from build123d import *

# Parameters (mm, degrees)
SKETCH_1_W           = 690
SKETCH_1_H           = 650
BOTTOM_PLATE_DEPTH   = 5
SKETCH_2_R           = 82.5
GRAB_CLEARANCE_DEPTH = 948.958332418
SKETCH_3_R           = 82.5
CUT_EXTRUDE_2_DEPTH  = 948.958332418
SKETCH_4_R           = 82.5
CUT_EXTRUDE_3_DEPTH  = 948.958332418
SKETCH_5_R           = 82.5
CUT_EXTRUDE_4_DEPTH  = 948.958332418


with BuildPart() as part:
    # 草图1 → Bottom_plate (new body)
    with BuildSketch(Plane.XY):
        with Locations((345, 325)):
            Rectangle(SKETCH_1_W, SKETCH_1_H)
    extrude(amount=BOTTOM_PLATE_DEPTH)

    # 草图2 → Grab_clearance (cut, through all)
    with BuildSketch(Plane.XY.offset(5)):
        with Locations((124, 92.5)):
            Circle(SKETCH_2_R)
    extrude(amount=-GRAB_CLEARANCE_DEPTH, mode=Mode.SUBTRACT)

    # 草图3 → 切除-拉伸2 (cut, through all)
    with BuildSketch(Plane.XY.offset(5)):
        with Locations((124, 557.5)):
            Circle(SKETCH_3_R)
    extrude(amount=-CUT_EXTRUDE_2_DEPTH, mode=Mode.SUBTRACT)

    # 草图4 → 切除-拉伸3 (cut, through all)
    with BuildSketch(Plane.XY.offset(5)):
        with Locations((566, 92.5)):
            Circle(SKETCH_4_R)
    extrude(amount=-CUT_EXTRUDE_3_DEPTH, mode=Mode.SUBTRACT)

    # 草图5 → 切除-拉伸4 (cut, through all)
    with BuildSketch(Plane.XY.offset(5)):
        with Locations((566, 557.5)):
            Circle(SKETCH_5_R)
    extrude(amount=-CUT_EXTRUDE_4_DEPTH, mode=Mode.SUBTRACT)


solid = part.part
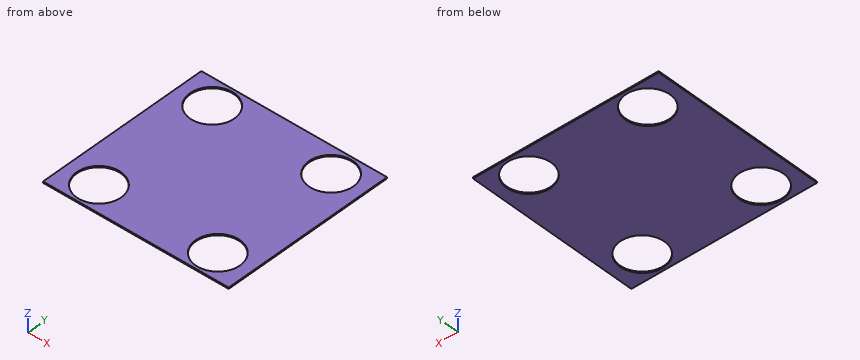
The listing builds one solid part. Answer for the finished solid, in the listing's coordinates (mm). Give positions to 0.01 mm unless a question says otherwise; leave off trailing zeros. Write each loop counter-clockwise with the first axis right and the second up, starting at its lowest first coordinate (ties: lowest second). Pieces come first, ordered by that corner, then holes.
1) Find the intervals of material crossed by L1, parallel to Y at x = 124, z = 2.75; L2, parallel to Y at x = 570, z = 2.95; L3, parallel to X at y = 78, z = 0.7, in increasing order.
2) Section C-C (y = 92.5) is taken. Write down the section's boundary in (x, z), and give its area (3 significant figures).
3) Given P1, Ø2, axis at y = 158.5, z = 3.5, coming from the -X side, flat-ended and moving along its own axis, determine where the tip first touches the part or whether it passes through.
4) Section A-A (z = 4.2) is taken. Write down the section's boundary in (x, y).
5) Section B-B (x = 124) is taken. Write down the section's boundary in (y, z), and give its area (3 significant figures).
Response:
1. L1: y = 0 to 10, 175 to 475, 640 to 650
1. L2: y = 0 to 10.1, 174.9 to 475.1, 639.9 to 650
1. L3: x = 0 to 42.78, 205.22 to 484.78, 647.22 to 690
2. outline: (0, 0) - (41.5, 0) - (41.5, 5) - (0, 5) - close; (206.5, 0) - (483.5, 0) - (483.5, 5) - (206.5, 5) - close; (648.5, 0) - (690, 0) - (690, 5) - (648.5, 5) - close
2. area: 1,800 mm2
3. P1: stops at x = 0
4. outline: (0, 0) - (690, 0) - (690, 650) - (0, 650) - close; hole circle Ø165 at (124, 92.5); hole circle Ø165 at (124, 557.5); hole circle Ø165 at (566, 92.5); hole circle Ø165 at (566, 557.5)
5. outline: (0, 0) - (10, 0) - (10, 5) - (0, 5) - close; (175, 0) - (475, 0) - (475, 5) - (175, 5) - close; (640, 0) - (650, 0) - (650, 5) - (640, 5) - close
5. area: 1,600 mm2
